Autodesk Inventor part; units mm, degrees
ref_plane "Start Plane" through (0, 0, 35.56) normal (0, 0, 1) x (1, 0, 0)
ref_plane "End Plane" through (0, 0, 495.3) normal (0, 0, 1) x (1, 0, 0)
ref_plane "Work Plane4" through (-716.28, -25.4, 568.96) normal (-0.6, 0, -0.8) x (-0.8, 0, 0.6)
ref_plane "Start Plane" through (0, 0, 35.56) normal (0, 0, 1) x (1, 0, 0)
ref_plane "End Plane" through (0, 0, 495.3) normal (0, 0, 1) x (1, 0, 0)
sketch "Sketch" plane through (0, 0, 0) normal (0, 0, 1) x (1, 0, 0)
  line L0 (-25.4, -25.4) -> (-25.4, 25.4)
  line L1 (-12.7, 38.1) -> (12.7, 38.1)
  line L2 (25.4, 25.4) -> (25.4, -25.4)
  line L3 (12.7, -38.1) -> (-12.7, -38.1)
  arc A0 (-25.4, -25.4) -> (-12.7, -38.1) centre (-12.7, -25.4) ccw
  arc A1 (-12.7, 38.1) -> (-25.4, 25.4) centre (-12.7, 25.4) ccw
  arc A2 (25.4, 25.4) -> (12.7, 38.1) centre (12.7, 25.4) ccw
  arc A3 (12.7, -38.1) -> (25.4, -25.4) centre (12.7, -25.4) ccw
  arc A4 (-12.7, 31.75) -> (-19.05, 25.4) centre (-12.7, 25.4) ccw
  line L4 (-12.7, 31.75) -> (12.7, 31.75)
  arc A5 (19.05, 25.4) -> (12.7, 31.75) centre (12.7, 25.4) ccw
  line L5 (19.05, 25.4) -> (19.05, -25.4)
  arc A6 (12.7, -31.75) -> (19.05, -25.4) centre (12.7, -25.4) ccw
  line L6 (12.7, -31.75) -> (-12.7, -31.75)
  arc A7 (-19.05, -25.4) -> (-12.7, -31.75) centre (-12.7, -25.4) ccw
  line L7 (-19.05, -25.4) -> (-19.05, 25.4)
  line L8 (0, 57.0224) -> (0, -57.0224) construction
  line L9 (-39.2424, 0) -> (39.2424, 0) construction
  dimension "d10" = 76.2
  dimension "d11" = 50.8
  dimension "d12" = 6.35
  dimension "d15" = 38.1
  dimension "d16" = 25.4
  dimension "d17" = 12.7
extrude "Body" add sketch "Sketch" along normal up to surface (459.74 mm away) from surface at 35.56
sketch "Sketch3" plane through (0, 0, 0) normal (0, 0, 1) x (1, 0, 0)
  line L0 (0, 0) -> (10, 0)
ref_plane "Work Plane3" through (0, 0, 0) normal (0, -1, 0) x (1, 0, 0)
ref_plane "Work Plane4" through (-716.28, -25.4, 568.96) normal (-0.6, 0, -0.8) x (-0.8, 0, 0.6)
split "Split1" plane through (-716.28, -25.4, 568.96) removes the side toward (-0.6, 0, -0.8)
ref_plane "Work Plane5" through (228.6, -25.4, 304.8) normal (0.6, 0, 0.8) x (0.8, 0, -0.6)
split "Split2" plane through (228.6, -25.4, 304.8) removes the side toward (0.6, 0, 0.8)
ref_plane "Work Plane6" through (223.52, 25.4, 340.36) normal (0.8, 0, -0.6) x (-0.6, 0, -0.8)
split "Split3" plane through (223.52, 25.4, 340.36) removes the side toward (0.8, 0, -0.6)
sketch "Sketch4" plane through (0, 0, 0) normal (0, -1, 0) x (1, 0, 0)
  line L0 (-2, 35.56) -> (12, 35.56)
  line L1 (-2, 495.3) -> (12, 495.3)
  dimension "d19" = 459.74
equation "\"d10\" = G_H"
equation "\"d11\" = G_W"
equation "\"d12\" = G_T"
equation "\"d15\" = 0.5 * d10"
equation "\"d16\" = 0.5 * d11"
equation "\"d17\" = G_IR"
equation "\"d3\" = G_L"
equation "\"G_W\" = 50.8"
equation "\"G_H\" = 76.2"
equation "\"G_T\" = 6.35"
equation "\"G_IR\" = 12.7"
equation "\"G_L\" = d19"
equation "\"G_OFFSET_START\" = -35.56"
equation "\"G_OFFSET_END\" = -12.7"
equation "\"d13\" = -G_OFFSET_START"
equation "\"d14\" = G_OFFSET_END + B_L"
equation "\"B_L\" = 508"
properties part number "AISC - 3 x 2 x 1/4 - 18.1" material "Steel, Mild"
Part model, mm, in its own coordinate system. A direction names the side the tool comes from. Round coordinates to 2 decimals unless told otherwise and drop trailing zeros. Write each loop counter-clockwise with the first axis right and the second up, starting at its lowest first coordinate (ties: lowest second). Pieces come first, ordered by that corner, then holes. Notation, with made-up numbers: M -22,68 L 17,68 A7 cw 17,74 Z; hole C 50.25,-6.5 d5. An arc over 180 degrees is marked long. One line per question, with ' | ' between items.
(1) Saw through at C-C on x = 1. Write the cut outline in (y, z).
Answer key:
outline: M -38.1,43.67 L -31.75,43.67 L -31.75,475.5 L -38.1,475.5 Z; M 31.75,43.67 L 38.1,43.67 L 38.1,475.5 L 31.75,475.5 Z
(2) Saw through at B-B on z = 408. Write the cut outline in (x, y).
Answer key:
outline: M -25.4,-25.4 A12.7 ccw -12.7,-38.1 L 12.7,-38.1 A12.7 ccw 25.4,-25.4 L 25.4,25.4 A12.7 ccw 12.7,38.1 L -12.7,38.1 A12.7 ccw -25.4,25.4 Z; hole M -19.05,-25.4 A6.35 ccw -12.7,-31.75 L 12.7,-31.75 A6.35 ccw 19.05,-25.4 L 19.05,25.4 A6.35 ccw 12.7,31.75 L -12.7,31.75 A6.35 ccw -19.05,25.4 Z
(3) Saw through at A-A on y = 2. Write the cut outline in (x, z), then the cut area to 3 significant figures.
Answer key:
outline: M -25.4,50.8 L -19.05,46.04 L -19.05,490.54 L -25.4,495.3 Z; M 19.05,67.73 L 25.4,76.2 L 25.4,457.2 L 19.05,461.96 Z | area: 5,280 mm^2
(4) 3-axis set-ups, long thin cutter, end or side, ignore diameter. For faces 1 (the face through (21.58, 34.48, 260.14)), 2 (the face through (-19.05, 0, 265)): which of +Z, -Z, +X, -X, +Y, -Y reach the whole face in a straight line?
Answer key:
face 1: +Z, -Z, +X, +Y | face 2: +Z, -Z
(5) Probe line 1 along X through (y, z) = (-25, 139); line 2 along Y through (x, z) = (9, 445); line 3 along X through (y, z) = (-12.5, 460.5). List the from-to ranges inside material, lowest first.
Answer key:
line 1: x = -25.4 to -19.05, 19.05 to 25.4 | line 2: y = -38.1 to -31.75, 31.75 to 38.1 | line 3: x = -25.4 to -19.05, 19.05 to 21
(6) Pin check, flat tips, straight feed: pin 1 (1 mm diameter, centred on x = 15.5, z = 215.5, fed in from -Y); pin 2 (3 mm diameter, centred on x = 6.5, y = -29.5, fed in from +Z); pin 3 (12 mm diameter, centred on x = 2, y = 26.5, fed in from +Z). Stop position of each tip, or through.
Answer key:
pin 1: stops at y = -37.89 | pin 2: passes through | pin 3: stops at z = 476.93
